Can you work these out from the model? Positions are in its coordinate system, mm. A direction names the side the tool comes from. Give positions to 0.01 mm unless a question says otherwise; leave off trailing zeros. Write each loop counter-clockwise with the first axis right and the second up, starting at its lowest first coordinate (ties: lowest second). Pieces come first, ordered by that corner, then holes.
1. Suppose I cut it at B-B (y = 67). Give the number of separate pieces and of enclosed holes in the cut face, and give its area (3 significant figures).
2. Thinking about a two-plate mould opening in Z: for faces 6 (the flat face through (6, 2, 23)), 7 (the cylindrical face through (4.975, 35.989, 16.247)), 8 (the cylindrical face through (-25.865, 0.986, 10.724)), which applies, pulls with the +Z half, pulls with the -Z half, needs draft (parallel to the pull), parting line crosses it, or undercut?
3. I'm going to push flat-ended pins straight in: pin 1 (1.5 mm diameter, centred on y = 23, z = -7.5, fed in from +X); pin 2 (10 mm diameter, centred on y = 36.5, z = -22, fed in from +X); pin 3 (5 mm diameter, centred on y = 29, z = -4.5, fed in from -X); pin 4 (17.5 mm diameter, centred on x = 0, z = 0, fed in from +Y). Where does each tip first touch, or does it pass through?
4. Suppose I cut it at A-A (x = 0). Please give me the cut outline in (y, z).
5. On a 3-axis mill with a long thin cutter (end or side, diameter ignored), from which of +Z, -Z, +X, -X, +Y, -Y can I reach the whole of each face in a straight line? I mean faces 1 (the cylindrical face through (-19.55, 35.99, 4.22)), 2 (the cylindrical face through (-2.994, 35.777, 22.804)), 3 (the flat face through (-3, 61, 10)), 4 (the flat face through (5, 73, 10.4)), 5 (the flat face through (-3, 11, -10)). Say none if no direction works.
6. If I drill on probe 1 along Z at (x, y) = (0, 1); probe 2 along X at (y, z) = (68, 0); probe 3 along Z at (x, y) = (0, 26.5), over which ranges is the centre line in solid material (lowest first)?
Autodesk Inventor part; units mm, degrees
ref_plane "YZ Plane" through (0, 0, 0) normal (1, 0, 0) x (0, 1, 0)
ref_plane "XZ Plane" through (0, 0, 0) normal (0, 1, 0) x (-1, 0, 0)
ref_plane "XY Plane" through (0, 0, 0) normal (0, 0, 1) x (1, 0, 0)
sketch "Sketch1" plane through (0, 0, 0) normal (0, 1, 0) x (-1, 0, 0)
  circle A0 centre (0, 0) radius 11.05
  circle A1 centre (0, 0) radius 28
  dimension "d0" = 22.1
  dimension "d1" = 56
extrude "Extrusion1" add sketch "Sketch1" along normal blind 2
sketch "Sketch2" plane through (0, 2, 0) normal (0, 1, 0) x (1, 0, 0)
  circle A0 centre (0, 0) radius 23
  dimension "d4" = 46
extrude "Extrusion2" add sketch "Sketch2" along normal blind 68
sketch "Sketch3" plane through (0, 70, 0) normal (0, 1, 0) x (1, 0, 0)
  circle A0 centre (0, 0) radius 23
extrude "Extrusion3" add sketch "Sketch3" along normal blind 3 draft 20
sketch "Sketch4" plane through (0, 2, 0) normal (0, -1, 0) x (1, 0, 0)
  circle A0 centre (0, 0) radius 11.05
extrude "Extrusion4" cut sketch "Sketch4" against normal blind 9
sketch "Sketch5" plane through (0, 11, 0) normal (0, -1, 0) x (1, 0, 0)
  circle A0 centre (0, 0) radius 10
  dimension "d11" = 20
extrude "Extrusion5" cut sketch "Sketch5" against normal up to next
sketch "Sketch6" plane through (0, 73, 0) normal (0, 1, 0) x (1, 0, 0)
  circle A0 centre (0, 0) radius 11.05
  dimension "d14" = 22.1
extrude "Extrusion6" cut sketch "Sketch6" against normal blind 12
sketch "Sketch7" plane through (0, 0, 0) normal (0, -1, 0) x (1, 0, 0)
  circle A0 centre (0, 0) radius 11.05
  circle A1 centre (0, 0) radius 28
  line L0 (0, 0) -> (43.5603, 0) construction
  line L1 (-10.3416, 8.6776) -> (-15.3209, 12.8558) construction
  arc A2 (-15.3019, 6.8128) -> (-16.75, 0) centre (0, 0) ccw construction
  arc A3 (-18.2709, 8.1347) -> (-20, 0) centre (0, 0) ccw
  arc A4 (-12.3329, 5.4909) -> (-13.5, 0) centre (0, 0) ccw
  arc A5 (-12.3329, 5.4909) -> (-18.2709, 8.1347) centre (-15.3019, 6.8128) ccw
  arc A6 (-20, 0) -> (-13.5, 0) centre (-16.75, 0) ccw
  arc A7 (-9.0333, -10.0325) -> (-13.3826, -14.8629) centre (-11.2079, -12.4477) ccw
  arc A8 (-6.1803, -19.0211) -> (-4.1717, -12.8393) centre (-5.176, -15.9302) ccw
  arc A9 (6.75, -11.6913) -> (10, -17.3205) centre (8.375, -14.5059) ccw
  arc A10 (16.1803, -11.7557) -> (10.9217, -7.9351) centre (13.551, -9.8454) ccw
  arc A11 (13.205, 2.8068) -> (19.563, 4.1582) centre (16.384, 3.4825) ccw
  arc A12 (16.1803, 11.7557) -> (10.9217, 7.9351) centre (13.551, 9.8454) ccw
  arc A13 (1.4111, 13.426) -> (2.0906, 19.8904) centre (1.7509, 16.6582) ccw
  arc A14 (-6.1803, 19.0211) -> (-4.1717, 12.8393) centre (-5.176, 15.9302) ccw
  arc A15 (-12.3329, 5.4909) -> (-13.5, 0) centre (0, 0) ccw
  arc A16 (-18.2709, 8.1347) -> (-20, 0) centre (0, 0) ccw
  arc A17 (-13.3826, -14.8629) -> (-6.1803, -19.0211) centre (0, 0) ccw
  arc A18 (-9.0333, -10.0325) -> (-4.1717, -12.8393) centre (0, 0) ccw
  arc A19 (10, -17.3205) -> (16.1803, -11.7557) centre (0, 0) ccw
  arc A20 (6.75, -11.6913) -> (10.9217, -7.9351) centre (0, 0) ccw
  arc A21 (13.205, 2.8068) -> (10.9217, 7.9351) centre (0, 0) ccw
  arc A22 (1.4111, 13.426) -> (-4.1717, 12.8393) centre (0, 0) ccw
  arc A23 (19.563, 4.1582) -> (16.1803, 11.7557) centre (0, 0) ccw
  arc A24 (2.0906, 19.8904) -> (-6.1803, 19.0211) centre (0, 0) ccw
  point P0 (-12.8312, 10.7667)
  point P1 (-14.2048, 8.8761)
  point P2 (-16.1011, 4.6169)
  point P3 (-16.587, 2.3311)
  dimension "d22" = 40
  dimension "d26" = 360
extrude "Extrusion7" cut sketch "Sketch7" against normal up to next contours A5 A4 A6 A3 | A18 A8 A17 A7 | A20 A10 A19 A9 | A21 A12 A23 A11 | A22 A14 A24 A13
fillet "Fillet1" radius 0.5 1 edges at (-23, 2, 0)
properties part number "spooler big"
Checks:
1. separate pieces: 1
1. enclosed holes: 6
1. area: 884 mm2
2. face 6: needs draft
2. face 7: undercut
2. face 8: parting line crosses it
3. pin 1: stops at x = 21.99
3. pin 2: stops at x = 15.49
3. pin 3: stops at x = -22.91
3. pin 4: passes through
4. outline: (0, -28) - (2, -28) - (2, -23.5) arc R0.5 cw to (2.5, -23) - (70, -23) - (73, -24.09) - (73, -11.05) - (61, -11.05) - (61, -10) - (11, -10) - (11, -11.05) - (0, -11.05) - close; (0, 11.05) - (11, 11.05) - (11, 10) - (61, 10) - (61, 11.05) - (73, 11.05) - (73, 13.5) - (0, 13.5) - close; (0, 20) - (73, 20) - (73, 24.09) - (70, 23) - (2.5, 23) arc R0.5 cw to (2, 23.5) - (2, 28) - (0, 28) - close
5. face 1: +Y, -Y
5. face 2: none
5. face 3: +Y
5. face 4: +Z, -Z, +X, -X, +Y
5. face 5: -Y
6. probe 1: z = -28 to -11.05, 11.05 to 13.5, 20 to 28
6. probe 2: x = -23 to -20, -13.5 to -11.05, 11.05 to 23
6. probe 3: z = -23 to -10, 10 to 13.5, 20 to 23
